Autodesk Inventor part; units mm, degrees
ref_plane "YZ Plane" through (0, 0, 0) normal (1, 0, 0) x (0, 1, 0)
ref_plane "XZ Plane" through (0, 0, 0) normal (0, 1, 0) x (-1, 0, 0)
ref_plane "XY Plane" through (0, 0, 0) normal (0, 0, 1) x (1, 0, 0)
sketch "Sketch1" plane through (0, 0, 0) normal (0, 0, 1) x (1, 0, 0)
  line L0 (28.0448, -41.9322) -> (-28.0448, -41.9322)
  line L1 (-28.0448, -41.9322) -> (-28.0448, 41.9322)
  line L2 (-28.0448, 41.9322) -> (28.0448, 41.9322)
  line L3 (28.0448, 41.9322) -> (28.0448, -41.9322)
  line L4 (28.0448, -41.9322) -> (-28.0448, 41.9322) construction
  line L5 (-28.0448, -41.9322) -> (28.0448, 41.9322) construction
  point P0 (0, 0)
  dimension "d0" = 56.0896
  dimension "d1" = 83.8645
extrude "Container Backplate" add sketch "Sketch1" along normal mid plane 1.5875
sketch "Sketch2" plane through (0, 0, -0.7937) normal (0, 0, -1) x (-1, 0, 0)
  line L0 (28.0448, 41.9322) -> (-28.0448, 41.9322)
  line L1 (-28.0448, 41.9322) -> (-28.0448, -41.9322)
  line L2 (-28.0448, -41.9322) -> (28.0448, -41.9322)
  line L3 (28.0448, -41.9322) -> (28.0448, 41.9322)
  line L4 (-29.6323, 43.5197) -> (29.6323, 43.5197)
  line L5 (29.6323, 43.5197) -> (29.6323, -43.5197)
  line L6 (29.6323, -43.5197) -> (-29.6323, -43.5197)
  line L7 (-29.6323, -43.5197) -> (-29.6323, 43.5197)
  line L8 (28.0448, 41.9322) -> (29.6323, 41.9322)
  line L9 (-28.0448, 41.9322) -> (-29.6323, 41.9322)
  point P0 (0, 0)
  point P1 (28.0448, 43.5197)
  point P2 (-28.0448, 43.5197)
  dimension "d4" = 1.5875
extrude "Container Walls" add sketch "Sketch2" against normal blind 11.7792 contours L8 L5 L6 L7 L9 L1 L2 L3
sketch "Sketch3" plane through (0, 0, 10.9855) normal (0, 0, 1) x (1, 0, 0)
  line L0 (-23.2823, -43.5197) -> (-20.1073, -43.5197)
  line L1 (-20.1073, -43.5197) -> (-20.1073, -40.3447)
  line L2 (-20.1073, -40.3447) -> (-23.2823, -40.3447)
  line L3 (-23.2823, -40.3447) -> (-23.2823, -43.5197)
  line L4 (-29.6323, -43.5197) -> (29.6323, -43.5197)
  line L5 (28.0448, -41.9322) -> (-28.0448, -41.9322)
  line L6 (-29.6323, 41.9322) -> (-29.6323, -43.5197)
  line L7 (-29.6323, 16.5322) -> (-26.4573, 16.5322)
  line L8 (-26.4573, 16.5322) -> (-26.4573, 13.3572)
  line L9 (-26.4573, 13.3572) -> (-29.6323, 13.3572)
  line L10 (-29.6323, 13.3572) -> (-29.6323, 16.5322)
  line L11 (28.0448, 41.9322) -> (-28.0448, 41.9322)
  line L12 (0, 41.9322) -> (0, -43.5197)
  line L13 (23.2823, -43.5197) -> (20.1073, -43.5197)
  line L14 (20.1073, -43.5197) -> (20.1073, -40.3447)
  line L15 (20.1073, -40.3447) -> (23.2823, -40.3447)
  line L16 (23.2823, -40.3447) -> (23.2823, -43.5197)
  line L17 (29.6323, 43.5197) -> (29.6323, -43.5197)
  line L18 (29.6323, 16.5322) -> (26.4573, 16.5322)
  line L19 (26.4573, 16.5322) -> (26.4573, 13.3572)
  line L20 (26.4573, 13.3572) -> (29.6323, 13.3572)
  line L21 (29.6323, 13.3572) -> (29.6323, 16.5322)
  point P0 (0, 0)
  point P1 (-29.6323, 43.5197)
  dimension "d7" = 3.175
  dimension "d8" = 3.175
  dimension "d9" = 6.35
  dimension "d10" = 3.175
  dimension "d11" = 3.175
  dimension "d12" = 25.4
extrude "Container Tabs" add sketch "Sketch3" along normal blind 0.7937 contours L3 L5 L1 L0 | L20 L19 L18 L17 | L6 L7 L8 L9 | L3 L2 L1 L5 | L14 L5 L16 L4 | L14 L15 L16 L5
sketch "Sketch11" plane through (0, 0, -0.7937) normal (0, 0, -1) x (-1, 0, 0)
  line L0 (-12.7381, 7.2803) -> (12.7381, 7.2803)
  line L1 (12.7381, 7.2803) -> (12.7381, 0.9303)
  line L2 (12.7381, 0.9303) -> (-12.7381, 0.9303)
  line L3 (-12.7381, 0.9303) -> (-12.7381, 7.2803)
  line L4 (-29.6323, -43.5197) -> (29.6323, -43.5197)
  point P0 (0, 0)
  point P1 (0, 7.2803)
  dimension "d58" = 25.4762
  dimension "d59" = 6.35
  dimension "d60" = 44.45
extrude "Servo Connector Tab" add sketch "Sketch11" along normal blind 44.45
properties part number "MovingCompartment"
CAD build for the part. Positions are in the model's coordinates, mm. A direction names the side the tool comes from. Give positions to 0.01 mm unless a question says otherwise; leave off trailing zeros. Write each loop counter-clockwise with the first axis right and the second up, starting at its lowest first coordinate (ties: lowest second). Pieces come first, ordered by that corner, then holes. Notation, with made-up numbers: (34, 31) -> (56, 31) arc R28 ccw to (56, 54) -> close; hole circle Ø2 at (-7.5, 42.25). An arc over 180 degrees is marked (long way). Return JSON: item names as keys, results as strings.
Item 1: Drill centre lines: probe 1 along X at (y, z) = (-9, 8); probe 2 along Z at (x, y) = (-1, 0); probe 3 along Y at (x, z) = (7.5, -8.5). Where is each one in solid material? Low to high.
Answer below:
{"probe 1": "x = -29.63 to -28.04, 28.04 to 29.63", "probe 2": "z = -0.79 to 0.79", "probe 3": "y = 0.93 to 7.28"}
Item 2: Two-plate mould, pull along X, no slides. Class faces 4 (the flat face through (-28, 15, 11.779)), 5 (the flat face through (-12.738, 4, -23)), 6 (the flat face through (0, 1, 0.794)): +X half, -X half, draft (parallel to the pull), parting line (faces both ways), or undercut.
Answer below:
{"face 4": "draft", "face 5": "-X half", "face 6": "undercut"}
Item 3: Band-saw the part on C-C (z = 8). List the corners of the cut face in (x, y).
Answer below:
{"outline": "(-29.63, -43.52) -> (29.63, -43.52) -> (29.63, 41.93) -> (28.04, 41.93) -> (28.04, -41.93) -> (-28.04, -41.93) -> (-28.04, 41.93) -> (-29.63, 41.93) -> close"}
Item 4: Drop flat-ended pins along their axis: pin 1 (0.6 mm diameter, centred on y = -42, z = 11.5, fed in from -X); pin 2 (1.7 mm diameter, centred on x = -5.5, y = -43, fed in from +Z); pin 3 (5 mm diameter, centred on x = -18, y = 24, fed in from -Z). Give the stop position or say it passes through.
Answer below:
{"pin 1": "stops at x = -23.28", "pin 2": "stops at z = 10.99", "pin 3": "stops at z = -0.79"}
Item 5: Tool access for faces 1 (the flat face through (0, 7.28, -23)), 2 (the flat face through (-29, -17, 10.986)), 3 (the flat face through (12.738, 4, -23)): list every direction of +Z, -Z, +X, -X, +Y, -Y with a clear straight run to the whole face (end or side of a thin tool).
Answer below:
{"face 1": "-Z, +X, -X, +Y", "face 2": "+Z, -X, -Y", "face 3": "-Z, +X, +Y, -Y"}
